```python
from build123d import *

# Parameters (mm, degrees)
BOSS_EXTRUDE1_DEPTH     = 20
CUT_EXTRUDE1_DEPTH      = 1
CUT_EXTRUDE1_DEPTH_BACK = 21


with BuildPart() as part:
    # Sketch1 → Boss-Extrude1 (new body)
    with BuildSketch(Plane.XY):
        with BuildLine():
            Line((-15, 15), (0, 15))
            Line((0, 15), (0, -15))
            Line((0, -15), (-15, -15))
            ThreePointArc((-15, -15), (-18.535533906, -13.535533906), (-20, -10))
            Line((-20, -10), (-20, 10))
            ThreePointArc((-20, 10), (-18.535533906, 13.535533906), (-15, 15))
        make_face()
    extrude(amount=BOSS_EXTRUDE1_DEPTH)

    # Sketch2 → Cut-Extrude1 (cut, two sides)
    with BuildSketch(Plane.XY.offset(20)) as cut_extrude1_sk:
        with BuildLine():
            ThreePointArc((-12.5, 0), (-10, -2.5), (-7.5, 0))
            Line((-7.5, 0), (-12.5, 0))
        make_face()
        with BuildLine():
            Line((-12.5, 0), (-7.5, 0))
            ThreePointArc((-7.5, 0), (-10, 2.5), (-12.5, 0))
        make_face()
    extrude(amount=CUT_EXTRUDE1_DEPTH, mode=Mode.SUBTRACT)
    extrude(cut_extrude1_sk.sketch, amount=-CUT_EXTRUDE1_DEPTH_BACK, mode=Mode.SUBTRACT)


solid = part.part
```
Work out the finished part from the listing and answer in its coordinate system (mm). Give positions to 0.01 mm unless a question says otherwise; leave off trailing zeros. Order: outer loops, then holes, each group sorted by start corner. A loop starts at its lowest first (then second) coordinate and runs counter-clockwise, first axis right, second up. Notation, with made-up numbers: (0.25, -33.75) -> (28.25, -33.75) arc R32 ccw to (28.25, -0.75) -> close; hole circle Ø8 at (28.25, 58). An arc over 180 degrees is marked (long way). Answer as CSV lines item,"result". Start each with the question number.
(1) Consider line 1 along Y through (x, z) = (-10, 11.25); line 2 along X through (y, z) = (-2, 9.25); line 3 along X through (y, z) = (-13.5, 6.75). Determine where each line is inside the solid, lowest interval first.
(2) Section C-C, the plane y = 0 is taken. Write down the section's boundary in (x, z), plus the area to 3 significant figures.
(3) Section B-B, the plane x = -10 is taken. Write down the section's boundary in (y, z), plus the area to 3 significant figures.
(4) This flat-tipped pin is pushed along its axis until it touches: pin 1 Ø1 at (x, z) = (-17, 9.5) entering from -Y. Where does it stop, or does it pass through?
(5) Section A-A, the plane z = 16.75 is taken. Write down the section's boundary in (x, y).
(6) Section D-D, the plane x = -16.75 is taken. Write down the section's boundary in (y, z), plus the area to 3 significant figures.
(7) For a pull along Y with two mould halves and no side action, classify faces 1 (the cylindrical face through (-19, 13, 10)), 2 (the cylindrical face through (-12.5, 0.1, 10.1)), 3 (the flat face through (-10, -3, 0)) as released by +Y, released by -Y, zero draft, split by the parting line, or undercut.
Entries:
1,line 1,"-15 to -2.5, 2.5 to 15"
1,line 2,"-20 to -11.5, -8.5 to 0"
1,line 3,"-18.57 to 0"
2,outline,"(-20, 0) -> (-12.5, 0) -> (-12.5, 20) -> (-20, 20) -> close; (-7.5, 0) -> (0, 0) -> (0, 20) -> (-7.5, 20) -> close"
2,area,"300 mm²"
3,outline,"(-15, 0) -> (-2.5, 0) -> (-2.5, 20) -> (-15, 20) -> close; (2.5, 0) -> (15, 0) -> (15, 20) -> (2.5, 20) -> close"
3,area,"500 mm²"
4,pin 1,"y = -14.77"
5,outline,"(-20, -10) arc R5 ccw to (-15, -15) -> (0, -15) -> (0, 15) -> (-15, 15) arc R5 ccw to (-20, 10) -> close; hole circle Ø5 at (-10, 0)"
6,outline,"(-14.68, 0) -> (14.68, 0) -> (14.68, 20) -> (-14.68, 20) -> close"
6,area,"587 mm²"
7,face 1,"released by +Y"
7,face 2,"undercut"
7,face 3,"zero draft"
